The listing builds one solid part. Answer for the finished solid, in the listing's coordinates (mm). Face numbers are marked on the shaded views. A direction names the side the tool comes from. Give positions to 0.01 mm unless a question says otherwise; leave off trailing zeros. Write each loop counter-clockwise with the first axis right and the second up, starting at its lowest first coordinate (ties: lowest second). Pieces come first, ordered by that corner, then holes. Notation, with made-up numbers: (82, 56.25) -> (119, 56.25) arc R12 cw to (119, 75.25) -> close; hole circle Ø10 at (51, -4.5). An arc over 180 degrees is marked (long way). One line per question, with ' | ' between items.
from build123d import *


with BuildPart() as part:
    # Main Shape Profile → Main Shape (revolve)
    with BuildSketch(Plane.XY, mode=Mode.PRIVATE) as main_shape_sk:
        Polygon((9.525, 44.45), (9.525, 25.4), (31.75, 25.4), (31.75, 15.24), (38.1, 15.24), (38.1, 8.89), (57.15, 8.89), (57.15, 0), (76.2, 0), (76.2, 44.45), align=None)
    revolve(main_shape_sk.sketch.rotate(Axis((0, 0, 0), (0, -1, 0)), 90), axis=Axis((0, 0, 0), (0, -1, 0)))


solid = part.part
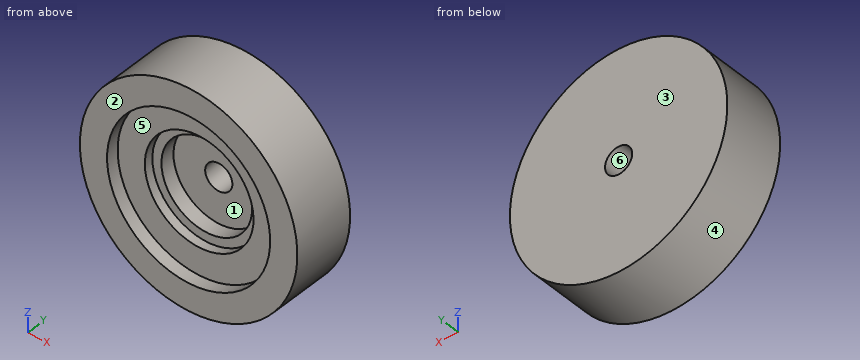
Item 1: A tool of negligible diameter and unlimited length cuts with its end or side. For the marked faces 1 and 2, from which of +Z, -Z, +X, -X, +Y, -Y can it reach the whole face along a straight path? Write none if from no direction.
Answers below:
face 1: -Y | face 2: +Z, -Z, +X, -X, -Y
Item 2: Find section B-B (z = 0). Write down the section's boundary in (x, y) (3 decimals).
Answers below:
outline: (-76.2, 0) -> (-57.15, 0) -> (-57.15, 8.89) -> (-38.1, 8.89) -> (-38.1, 15.24) -> (-31.75, 15.24) -> (-31.75, 25.4) -> (-9.525, 25.4) -> (-9.525, 44.45) -> (-76.2, 44.45) -> close; (9.525, 25.4) -> (31.75, 25.4) -> (31.75, 15.24) -> (38.1, 15.24) -> (38.1, 8.89) -> (57.15, 8.89) -> (57.15, 0) -> (76.2, 0) -> (76.2, 44.45) -> (9.525, 44.45) -> close
Item 3: Find section C-C (y = 12.5). Write down the section's boundary in (x, z), then the cut area to 3 significant figures.
Answers below:
outline: circle Ø152.4 at (0, 0); hole circle Ø76.2 at (0, 0) | area: 13,700 mm²
Item 4: Find section D-D (z = 23). Write down the section's boundary in (x, y), then the cut area to 3 significant figures.
Answers below:
outline: (-72.65, 0) -> (-52.32, 0) -> (-52.32, 8.89) -> (-30.37, 8.89) -> (-30.37, 15.24) -> (-21.89, 15.24) -> (-21.89, 25.4) -> (21.89, 25.4) -> (21.89, 15.24) -> (30.37, 15.24) -> (30.37, 8.89) -> (52.32, 8.89) -> (52.32, 0) -> (72.65, 0) -> (72.65, 44.45) -> (-72.65, 44.45) -> close | area: 4,700 mm²
Item 5: Flat-ended cylindrical pins translate along their axes: pin 1 (2 mm diameter, centred on x = -14.5, y = 38.5, fed in from +Z); pin 2 (6 mm diameter, centred on x = -40, y = 23, fed in from +Z); pin 3 (10 mm diameter, centred on y = 31, z = -31, fed in from +X). Find the tip coordinate at first contact, or state that the pin passes through.
Answers below:
pin 1: z = 74.99 | pin 2: z = 66.61 | pin 3: x = 71.63
Item 6: Determine the mould class of the marked faces 3, 4, 5 and 6 for opening direction X: pulls with the +X half, pulls with the -X half, needs draft (parallel to the pull), parting line crosses it, or undercut.
Answers below:
face 3: needs draft | face 4: parting line crosses it | face 5: undercut | face 6: undercut
Item 7: Find section A-A (x = 0). Write down the section's boundary in (y, z) (3 decimals).
Answers below:
outline: (0, -76.2) -> (44.45, -76.2) -> (44.45, -9.525) -> (25.4, -9.525) -> (25.4, -31.75) -> (15.24, -31.75) -> (15.24, -38.1) -> (8.89, -38.1) -> (8.89, -57.15) -> (0, -57.15) -> close; (0, 57.15) -> (8.89, 57.15) -> (8.89, 38.1) -> (15.24, 38.1) -> (15.24, 31.75) -> (25.4, 31.75) -> (25.4, 9.525) -> (44.45, 9.525) -> (44.45, 76.2) -> (0, 76.2) -> close
Item 8: Consider line 1 (X direction, y = 37.5, z = -0.5); line 2 (X direction, y = 10.5, z = 0); line 3 (Y direction, x = 33.5, z = 7). Determine where each line is inside the solid, lowest interval first. Write a range as [from, to].
Answers below:
line 1: [-76.2, -9.51], [9.51, 76.2] | line 2: [-76.2, -38.1], [38.1, 76.2] | line 3: [15.24, 44.45]
